The figure shows three views and two pictorial views of one solid part (mm, origin at its lowest corner). Answer the questions. Give positions to 0.01 mm unless a question says otherwise; leave off trailing zeros. Write each loop counter-clockwise with the first axis right and the second up, starting at its lowest first coordinate (ties: lowest second). Pieces come first, ordered by that corner, then holes. Notation, with made-up numbers: (33.25, 39) -> (69.25, 39) arc R11 cw to (69.25, 56) -> close; hole circle Ø10 at (46, -29). An arc over 180 degrees is marked (long way). Use a Markdown table: item, result.
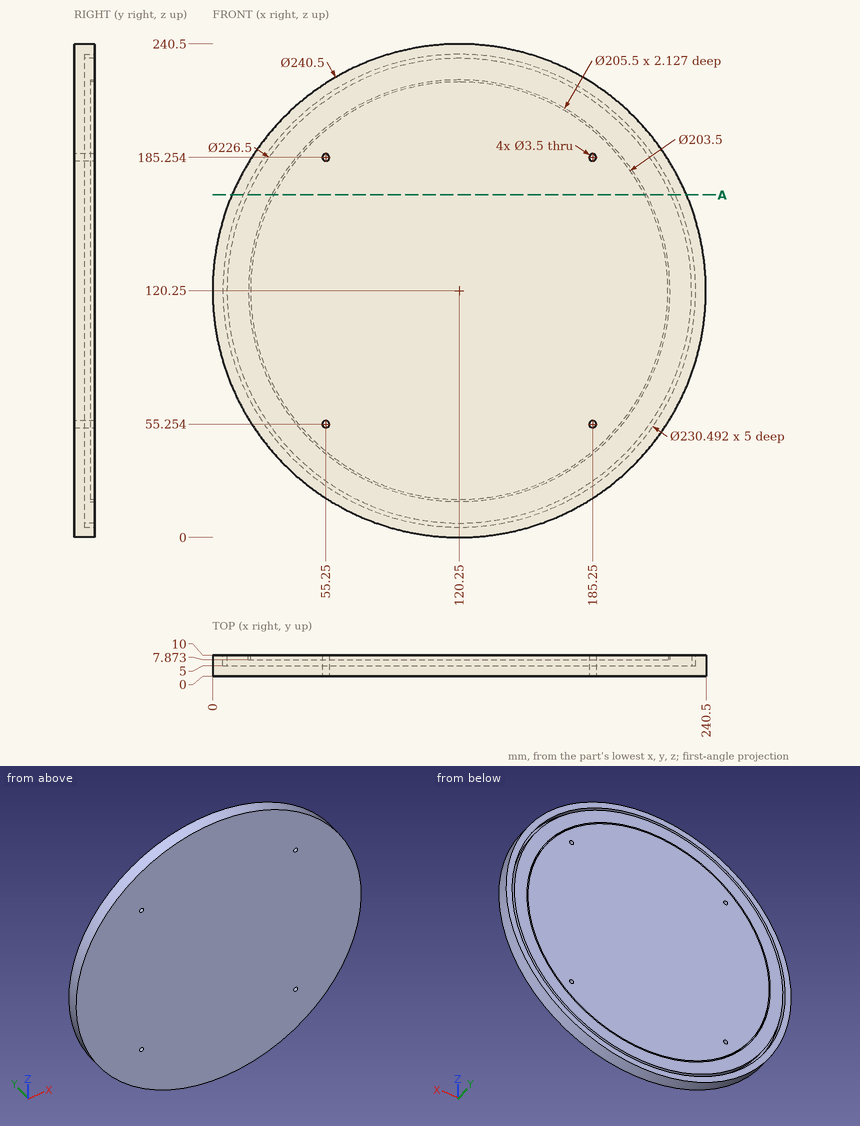
Item 1: A cutting plane is placed at A-A (z = 167). Give the vertices of the cut face in (x, y), then the cut area to 3 significant figures.
Return value:
| item | result |
|---|---|
| outline | (9.46, 0) -> (231.04, 0) -> (231.04, 10) -> (225.59, 10) -> (225.59, 5) -> (223.4, 5) -> (223.4, 10) -> (211.75, 10) -> (211.75, 7.87) -> (210.62, 7.87) -> (210.62, 10) -> (29.88, 10) -> (29.88, 7.87) -> (28.75, 7.87) -> (28.75, 10) -> (17.1, 10) -> (17.1, 5) -> (14.91, 5) -> (14.91, 10) -> (9.46, 10) -> close |
| area | 2,190 mm^2 |
Item 2: Straight lines are drawn through the part: line 1 along Z through (x, y) = (119, 6); line 2 along Z through (x, y) = (112, 7.5); line 3 along X through (y, z) = (9.5, 50.5) (1 decimal). For each, find the intervals that lie inside material, in ascending order. Write a range as [from, to].
Return value:
| item | result |
|---|---|
| line 1 | [0.01, 5.01], [7.01, 233.49], [235.49, 240.49] |
| line 2 | [0.28, 5.3], [7.3, 233.2], [235.2, 240.22] |
| line 3 | [22.3, 28.5], [31, 44.8], [46.2, 194.3], [195.7, 209.5], [212, 218.2] |
Item 3: Each of these flat-tipped pins is pushed along its axis until it touches: P1, Ø5, axis at x = 93, y = 6, coming from the -Z side (1 decimal); P2, Ø5, axis at x = 141, y = 7, coming from the +Z side; P3, Ø4.5, axis at x = 55.25, z = 55.25, coming from the -Y side; P4, Ø3, axis at y = 3.5, z = 151.5, coming from the +X side. Where does it stop, or does it pass through?
Return value:
| item | result |
|---|---|
| P1 | z = 2.6 |
| P2 | z = 239.11 |
| P3 | y = 0 |
| P4 | x = 236.76 |
